Input: part model. Units: mm. Frame: model coordinates. A direction names the side the tool comes from. Coordinates: 2 decimals unless noted, no trailing zeros. Loops run counter-clockwise (first coordinate to the right, second up) from the corner with the lowest first, then second, coordinate; pieces in that order, holes last.
(1) Section B-B, the plane y = 0. Return loops of the section in (x, z), then the cut area to 3 significant figures.
(2) Mould query, pull axis X, two halves, no side actions, for faces 4 (the face through (4.101, 31.232, 8.986)), 5 (the face through (-27, -17, 8)), 6 (the face through (10, -22.6, 3.7)), 7 (the face through (-13.71, 21.5, 7.04)). Classes: released by +X, released by -X, zero draft, split by the parting line, or undercut.
(3) Section C-C, the plane x = -23. Return loops of the section in (y, z), then the cut area to 3 significant figures.
(4) Contact query for flat-ended pins moving along their axis: P1, Ø3, axis at x = -10.5, z = 5, coming from the +Y side; P2, Ø1.5, axis at x = 3, y = 10, coming from the +Z side; P3, Ø1, axis at x = -21.5, z = 5, coming from the -Y side. Output: stop coordinate, or through.
(5) Line query: L1, parallel to Y at x = 0, z = 8.5; L2, parallel to Y at x = 0, z = 5.7; L3, parallel to Z at x = -5, y = -17.5. Output: solid intervals per line, ascending.
(6) Section A-A, the plane x = 0. Return loops of the section in (y, z), then the cut area to 3 significant figures.
(7) Section D-D, the plane z = 9. Return loops of the section in (x, y).
(8) Set-up query: faces 1 (the face through (0, -31, 7.5)), 2 (the face through (0, 1, 4)), 3 (the face through (29.11, 26.7, 3.94)). Return all of +Z, -Z, +X, -X, +Y, -Y with unobstructed straight access to the full face (end or side cutting, diameter ignored); none if empty.
```python
from build123d import *

# Parameters (mm, degrees)
F2_W     = 8
F2_H     = 0.65
F3_DEPTH = 3.5
F4_DEPTH = 2.6


with BuildPart() as f1:
    # F0 (on Front) → F1 (revolve)
    with BuildSketch(Plane.XZ):
        Polygon((-39.5, 8), (-39.5, 0), (0, 0), (0, 4), (-25.5, 4), (-25.5, 10), (-31.5, 10), (-31.5, 8), align=None)
    revolve(axis=Axis((0, 0, 4.935035), (0, 0, -1)))

    # F2 (on face) → F3 (cut)
    with BuildSketch(Plane.XY.offset(4)):
        with Locations((0, -39.175)):
            Rectangle(F2_W, F2_H)
        Polygon((4, -38.8), (4, -38.5), (-4, -38.5), (-4, -38.85), (4, -38.85), align=None)
        with BuildLine():
            Line((10, -23.457408), (10, -2.5))
            Line((10, -2.5), (-10, -2.5))
            Line((-10, -2.5), (-10, -23.457408))
            ThreePointArc((-10, -23.457408), (0, -25.5), (10, -23.457408))
        make_face()
        with BuildLine():
            Line((10, -35), (10, -23.457408))
            ThreePointArc((10, -23.457408), (0, -25.5), (-10, -23.457408))
            Line((-10, -23.457408), (-10, -35))
            Line((-10, -35), (-6, -38.5))
            Line((-6, -38.5), (-4, -38.5))
            Line((-4, -38.5), (4, -38.5))
            Line((4, -38.5), (6, -38.5))
            Line((6, -38.5), (10, -35))
        make_face()
    extrude(amount=F3_DEPTH, mode=Mode.SUBTRACT)

    # F2 (on face) → F4 (cut)
    with BuildSketch(Plane.XY.offset(4)):
        with BuildLine():
            Line((10, -23.457408), (10, -2.5))
            Line((10, -2.5), (-10, -2.5))
            Line((-10, -2.5), (-10, -23.457408))
            ThreePointArc((-10, -23.457408), (0, -25.5), (10, -23.457408))
        make_face()
        with BuildLine():
            Line((10, -35), (10, -23.457408))
            ThreePointArc((10, -23.457408), (0, -25.5), (-10, -23.457408))
            Line((-10, -23.457408), (-10, -35))
            Line((-10, -35), (-6, -38.5))
            Line((-6, -38.5), (-4, -38.5))
            Line((-4, -38.5), (4, -38.5))
            Line((4, -38.5), (6, -38.5))
            Line((6, -38.5), (10, -35))
        make_face()
    extrude(amount=-F4_DEPTH, mode=Mode.SUBTRACT)


solid = f1.part
```
Report:
1. outline: (-39.5, 0) - (39.5, 0) - (39.5, 8) - (31.5, 8) - (31.5, 10) - (25.5, 10) - (25.5, 4) - (-25.5, 4) - (-25.5, 10) - (-31.5, 10) - (-31.5, 8) - (-39.5, 8) - close
1. area: 452 mm2
2. face 4: split by the parting line
2. face 5: zero draft
2. face 6: undercut
2. face 7: undercut
3. outline: (-32.11, 0) - (32.11, 0) - (32.11, 8) - (21.52, 8) - (21.52, 10) - (11.01, 10) - (11.01, 4) - (-11.01, 4) - (-11.01, 10) - (-21.52, 10) - (-21.52, 8) - (-32.11, 8) - close
3. area: 468 mm2
4. P1: stops at y = 38.46
4. P2: stops at z = 4
4. P3: stops at y = -33.46
5. L1: y = -31.5 to -25.5, 25.5 to 31.5
5. L2: y = 25.5 to 39.5
5. L3: z = 0 to 1.4
6. outline: (-39.5, 0) - (39.5, 0) - (39.5, 8) - (31.5, 8) - (31.5, 10) - (25.5, 10) - (25.5, 4) - (-2.5, 4) - (-2.5, 1.4) - (-38.5, 1.4) - (-38.5, 4) - (-39.5, 4) - close; (-39.5, 7.5) - (-25.5, 7.5) - (-25.5, 10) - (-31.5, 10) - (-31.5, 8) - (-39.5, 8) - close
6. area: 309 mm2
7. outline: circle Ø63 at (0, 0); hole circle Ø51 at (0, 0)
8. face 1: none
8. face 2: +Z
8. face 3: +Z, -Z
